from build123d import *

# Parameters (mm, degrees)
SKETCH_1_R          = 5
EXTRUDE_1_DEPTH     = 93
SKETCH_2_R          = 6
EXTRUDE_2_DEPTH     = 3
SKETCH_3_R          = 15
SKETCH_3_R_2        = 2
EXTRUDE_3_DEPTH     = 3
SKETCH_6_R          = 2
CUT_EXTRUDE_3_DEPTH = 102.247222184
SKETCH_7_R          = 3
CUT_EXTRUDE_4_DEPTH = 3


with BuildPart() as part:
    # 草图1 → 凸台-拉伸1 (new body)
    with BuildSketch(Plane.XY):
        with Locations(Location((0, 0, 0), (0, 0, 180))):
            Circle(SKETCH_1_R)
    extrude(amount=EXTRUDE_1_DEPTH)

    # 草图2 → 凸台-拉伸2 (add)
    with BuildSketch(Plane.XY.offset(93)):
        Circle(SKETCH_2_R)
    extrude(amount=EXTRUDE_2_DEPTH)

    # 草图3 → 凸台-拉伸3 (add)
    with BuildSketch(Plane.XY.offset(96)):
        Circle(SKETCH_3_R)
        with Locations((0, 10)):
            Circle(SKETCH_3_R_2, mode=Mode.SUBTRACT)
        with Locations((10, 0)):
            Circle(SKETCH_3_R_2, mode=Mode.SUBTRACT)
        with Locations((0, -10)):
            Circle(SKETCH_3_R_2, mode=Mode.SUBTRACT)
        with Locations((-10, 0)):
            Circle(SKETCH_3_R_2, mode=Mode.SUBTRACT)
        with Locations((7.071067812, 7.071067812)):
            Circle(SKETCH_3_R_2, mode=Mode.SUBTRACT)
        with Locations((7.071067812, -7.071067812)):
            Circle(SKETCH_3_R_2, mode=Mode.SUBTRACT)
        with Locations((-7.071067812, -7.071067812)):
            Circle(SKETCH_3_R_2, mode=Mode.SUBTRACT)
        with Locations((-7.071067812, 7.071067812)):
            Circle(SKETCH_3_R_2, mode=Mode.SUBTRACT)
    extrude(amount=EXTRUDE_3_DEPTH)

    # 草图6 → 切除-拉伸3 (cut, through all)
    with BuildSketch(Plane(origin=(0, 0, 0), x_dir=(-1, 0, 0), z_dir=(0, 0, -1))):
        Circle(SKETCH_6_R)
    extrude(amount=-CUT_EXTRUDE_3_DEPTH, mode=Mode.SUBTRACT)

    # 草图7 → 切除-拉伸4 (cut)
    with BuildSketch(Plane.XY.offset(99)):
        Circle(SKETCH_7_R)
    extrude(amount=-CUT_EXTRUDE_4_DEPTH, mode=Mode.SUBTRACT)


solid = part.part
The model under review builds one solid part; all positions refer to its coordinate system, in mm. A direction names the side the tool comes from. Round coordinates to 2 decimals unless told otherwise and drop trailing zeros. Loops run counter-clockwise (first coordinate to the right, second up) from the corner with the lowest first, then second, coordinate; pieces in that order, holes last. Notation, with made-up numbers: (86, 1) -> (107, 1) arc R12 cw to (107, 23) -> close; hole circle Ø3 at (22, -1.5). An arc over 180 degrees is marked (long way). Return JSON: item names as keys, results as strings.
(1) For line 1 (Y direction, x = 0.25, z = 41.5); line 2 (Y direction, x = 0, z = 96.9); line 3 (Z direction, x = -3, y = 6), list the stretches that pass through material, from the lowest coordinate up.
Solved:
{"line 1": "-4.99 to -1.98, 1.98 to 4.99", "line 2": "-15 to -12, -8 to -3, 3 to 8, 12 to 15", "line 3": "96 to 99"}
(2) Add section D-D on z = 44. Write out the cut boundary in (x, y).
Solved:
{"outline": "circle Ø10 at (0, 0); hole circle Ø4 at (0, 0)"}
(3) Add section B-B on y = 10. Write out the cut boundary in (x, z).
Solved:
{"outline": "(-11.18, 96) -> (-2, 96) -> (-2, 99) -> (-11.18, 99) -> close; (2, 96) -> (11.18, 96) -> (11.18, 99) -> (2, 99) -> close"}
(4) Add section A-A on x = 0. Write out the cut boundary in (y, z).
Solved:
{"outline": "(-15, 96) -> (-12, 96) -> (-12, 99) -> (-15, 99) -> close; (-8, 96) -> (-6, 96) -> (-6, 93) -> (-5, 93) -> (-5, 0) -> (-2, 0) -> (-2, 96) -> (-3, 96) -> (-3, 99) -> (-8, 99) -> close; (2, 0) -> (5, 0) -> (5, 93) -> (6, 93) -> (6, 96) -> (8, 96) -> (8, 99) -> (3, 99) -> (3, 96) -> (2, 96) -> close; (12, 96) -> (15, 96) -> (15, 99) -> (12, 99) -> close"}
(5) For pin 1 (5 mm diameter, centred on y = -3, z = 73.5, fed in from +X); pin 2 (1 mm diameter, centred on y = 1.5, z = 82, fed in from -X); pin 3 (6 mm diameter, centred on y = -4.5, z = 23.5, fed in from -X); pin 4 (3.5 mm diameter, centred on x = 7.07, y = -7.07, fed in from -Z), all flat-tipped, find the tip position at first contact; note any pin that passes through.
Solved:
{"pin 1": "x = 4.97", "pin 2": "x = -4.9", "pin 3": "x = -4.77", "pin 4": "through"}
(6) For faces 4 (the cylindrical face through (-6, 0, 94)), 5 (the cylindrical face through (-3, 0, 98)), 6 (the cylindrical face through (-6, -5.38, 97.48)), list the 3-axis set-ups (+Z, -Z, +X, -X, +Y, -Y) from which the entire face can be reached by the end or side of a thin tool; tool diameter is ignored.
Solved:
{"face 4": "-Z", "face 5": "+Z", "face 6": "+Z, -Z"}
(7) The part is to be moulded in two halves that separate along Y. For faces 1 (the cylindrical face through (-14.985, 0.66, 97.479)), 2 (the cylindrical face through (8.4, -1.2, 97.5)), 3 (the flat face through (-4, 4, 93)), say which applies: released by +Y, released by -Y, zero draft, split by the parting line, or undercut.
Solved:
{"face 1": "split by the parting line", "face 2": "undercut", "face 3": "zero draft"}
